Check sheet for the modelled part. Datum: model origin and axes. Units: mm. Give positions to 0.01 mm unless a question says otherwise; leave off trailing zeros. Write each loop counter-clockwise with the first axis right and the second up, starting at its lowest first coordinate (ties: lowest second). Pieces come first, ordered by that corner, then holes. Notation, with made-up numbers: (-10.75, -20.5) -> (23.25, -20.5) arc R21 cw to (23.25, -7.5) -> close; hole circle Ø8 at (17, 8.5). An arc over 180 degrees is marked (long way). Answer as a JSON object with one key per item and string values.
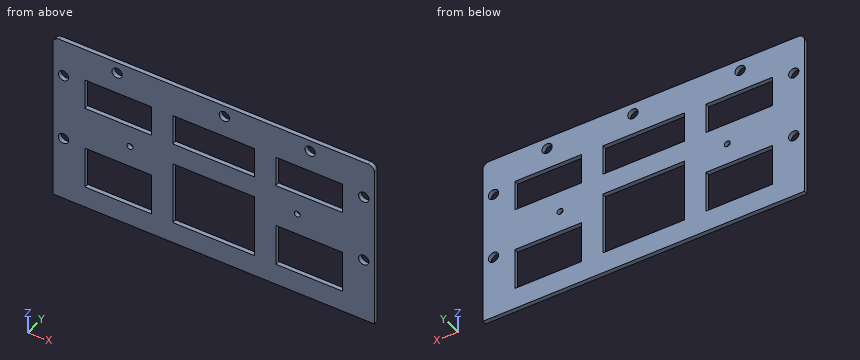
from build123d import *

# Parameters (mm, degrees)
ESQUISSE1_W        = 150
ESQUISSE1_H        = 79.06
ESQUISSE1_R        = 2.4
ESQUISSE1_R_2      = 1.4
ESQUISSE1_W_2      = 31
ESQUISSE1_H_2      = 19.53
ESQUISSE1_W_3      = 38
ESQUISSE1_H_3      = 29.53
ESQUISSE1_H_4      = 14.26
BOSS_EXTRU_1_DEPTH = 2
CONG_1_R           = 3


with BuildPart() as part:
    # Esquisse1 → Boss.-Extru.1 (new body)
    with BuildSketch(Plane(origin=(0, 0, 0), x_dir=(1, 0, 0), z_dir=(0, 1, 0))):
        with Locations((75, 39.53)):
            Rectangle(ESQUISSE1_W, ESQUISSE1_H)
        with Locations(Location((5, 49.04, 0), (0, 0, 270))):
            Circle(ESQUISSE1_R, mode=Mode.SUBTRACT)
        with Locations(Location((5, 17.48, 0), (0, 0, 270))):
            Circle(ESQUISSE1_R, mode=Mode.SUBTRACT)
        with Locations(Location((29.99, 5.27, 0), (0, 0, 270))):
            Circle(ESQUISSE1_R, mode=Mode.SUBTRACT)
        with Locations(Location((80, 5.27, 0), (0, 0, 270))):
            Circle(ESQUISSE1_R, mode=Mode.SUBTRACT)
        with Locations(Location((120.01, 5.27, 0), (0, 0, 270))):
            Circle(ESQUISSE1_R, mode=Mode.SUBTRACT)
        with Locations(Location((145, 49.04, 0), (0, 0, 270))):
            Circle(ESQUISSE1_R, mode=Mode.SUBTRACT)
        with Locations(Location((145, 17.48, 0), (0, 0, 270))):
            Circle(ESQUISSE1_R, mode=Mode.SUBTRACT)
        with Locations(Location((36, 39.53, 0), (0, 0, 270))):
            Circle(ESQUISSE1_R_2, mode=Mode.SUBTRACT)
        with Locations(Location((114, 39.53, 0), (0, 0, 270))):
            Circle(ESQUISSE1_R_2, mode=Mode.SUBTRACT)
        with Locations((30.5, 59.295)):
            Rectangle(ESQUISSE1_W_2, ESQUISSE1_H_2, mode=Mode.SUBTRACT)
        with Locations((75, 54.295)):
            Rectangle(ESQUISSE1_W_3, ESQUISSE1_H_3, mode=Mode.SUBTRACT)
        with Locations((119.5, 59.295)):
            Rectangle(ESQUISSE1_W_2, ESQUISSE1_H_2, mode=Mode.SUBTRACT)
        with Locations((119.5, 22.4)):
            Rectangle(ESQUISSE1_W_2, ESQUISSE1_H_4, mode=Mode.SUBTRACT)
        with Locations((75, 22.4)):
            Rectangle(ESQUISSE1_W_3, ESQUISSE1_H_4, mode=Mode.SUBTRACT)
        with Locations((30.5, 22.4)):
            Rectangle(ESQUISSE1_W_2, ESQUISSE1_H_4, mode=Mode.SUBTRACT)
    extrude(amount=BOSS_EXTRU_1_DEPTH)

    # Congé1
    cong_1_edges = [part.edges().sort_by_distance(p)[0] for p in [
        (150, 1, 0),
        (0, 1, 0),
    ]]
    fillet(cong_1_edges, radius=CONG_1_R)


solid = part.part
1. Sectioned sample at A-A, the plane x = 120.01. Enter the section's corners in (y, z), plus the area to 3 significant figures.
Determined:
{"outline": "(0, -79.06) -> (2, -79.06) -> (2, -69.06) -> (0, -69.06) -> close; (0, -49.53) -> (2, -49.53) -> (2, -29.53) -> (0, -29.53) -> close; (0, -15.27) -> (2, -15.27) -> (2, -7.67) -> (0, -7.67) -> close; (0, -2.87) -> (2, -2.87) -> (2, 0) -> (0, 0) -> close", "area": "80.9 mm^2"}
2. Sectioned sample at B-B, the plane z = -17.48. Enter the section's corners in (x, y).
Determined:
{"outline": "(0, 0) -> (2.6, 0) -> (2.6, 2) -> (0, 2) -> close; (7.4, 0) -> (15, 0) -> (15, 2) -> (7.4, 2) -> close; (46, 0) -> (56, 0) -> (56, 2) -> (46, 2) -> close; (94, 0) -> (104, 0) -> (104, 2) -> (94, 2) -> close; (135, 0) -> (142.6, 0) -> (142.6, 2) -> (135, 2) -> close; (147.4, 0) -> (150, 0) -> (150, 2) -> (147.4, 2) -> close"}
3. Sectioned sample at C-C, the plane z = -42.5. Enter the section's corners in (x, y), plus the area to 3 significant figures.
Determined:
{"outline": "(0, 0) -> (56, 0) -> (56, 2) -> (0, 2) -> close; (94, 0) -> (150, 0) -> (150, 2) -> (94, 2) -> close", "area": "224 mm^2"}
4. Go/stop test with a flat-tipped pin: P1, Ø1.7, axis at x = 36, z = -39.53, coming from the -Y side. Record where the tip stops, or that it passes through.
Determined:
{"P1": "through"}
5. Scan lines: L1, parallel to X at y = 1.5, z = -21.5; L2, parallel to Z at x = 21.5, y = 0.65; L3, parallel to X at y = 1.9, z = -49. Record each from-to range of solid material in increasing order. Write a range as [from, to].
Determined:
{"L1": "[0, 15], [46, 56], [94, 104], [135, 150]", "L2": "[-79.06, -69.06], [-49.53, -29.53], [-15.27, 0]", "L3": "[0, 2.6], [7.4, 56], [94, 142.6], [147.4, 150]"}
6. Sectioned sample at D-D, the plane x = 36. Enter the section's corners in (y, z).
Determined:
{"outline": "(0, -79.06) -> (2, -79.06) -> (2, -69.06) -> (0, -69.06) -> close; (0, -49.53) -> (2, -49.53) -> (2, -40.93) -> (0, -40.93) -> close; (0, -38.13) -> (2, -38.13) -> (2, -29.53) -> (0, -29.53) -> close; (0, -15.27) -> (2, -15.27) -> (2, 0) -> (0, 0) -> close"}
